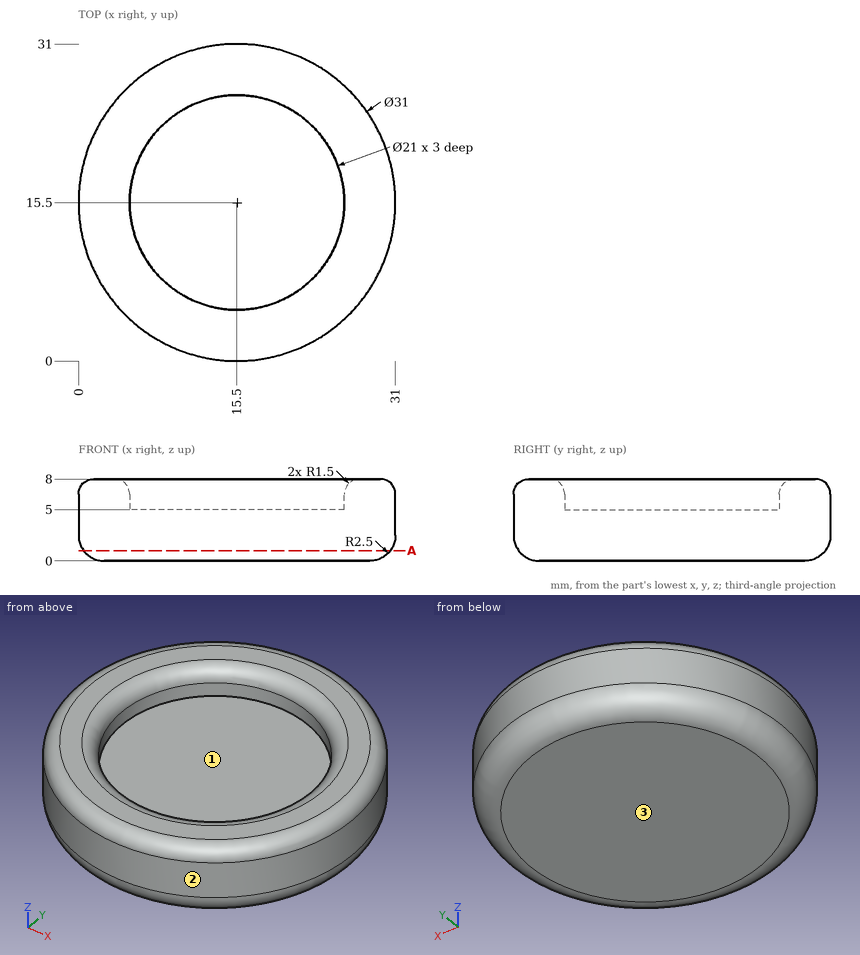
The drawing under review shows one solid part. Ordinate dimensions are in mm from its lowest x, y, z. Round coordinates to 2 decimals unless told otherwise and drop trailing zeros. Write each loop counter-clockwise with the first axis right and the second up, starting at its lowest first coordinate (ties: lowest second). Pieces come first, ordered by that corner, then holes.
(1) Wall thickness on L1, parallel to Y at x = 15.5, z = 5.8; L2, parallel to Y at x = 19.5, z = 5.75; L3, parallel to Z at x = 21, y = 12.5: over which ranges is each line inside the solid? List them lowest first.
(2) Mouldability with a two-part tool opening along X and no side actions: class the marked faces 1, 2 and 3 as +X half, -X half, draft (parallel to the pull), parting line (faces both ways), or undercut.
(3) Insertion check: pin 1 (6 mm diameter, centred on x = 15.5, y = 4.5, fed in from +Z); pin 2 (4 mm diameter, centred on x = 11.5, z = 6, fed in from +Y); pin 3 (1 mm diameter, centred on y = 13, z = 6, fed in from -X); pin 4 (3 mm diameter, centred on y = 23, z = 1.5, fed in from +X). Each pin has a flat end and moves straight along its axis. Give the tip position at first contact, or say it passes through.
(4) We need section A-A on z = 1. Give the boundary of the cut face in (x, y).
Findings below:
1. L1: y = 0 to 5, 26 to 31
1. L2: y = 0.53 to 5.79, 25.21 to 30.47
1. L3: z = 0 to 5
2. face 1: undercut
2. face 2: parting line
2. face 3: draft
3. pin 1: stops at z = 8
3. pin 2: stops at y = 30.87
3. pin 3: stops at x = 0.13
3. pin 4: stops at x = 29.7
4. outline: circle Ø30 at (15.5, 15.5)
